Part model, mm, in its own coordinate system. A direction names the side the tool comes from. Give positions to 0.01 mm unless a question says otherwise; leave off trailing zeros. Order: outer loops, then holes, each group sorted by start corner. A loop starts at its lowest first (then second) coordinate and runs counter-clockwise, first axis right, second up. Notation, with made-up numbers: (-27, 73.5) - (15, 73.5) arc R7 ccw to (15, 85.5) - close; hole circle Ø10 at (63, 19.25). An arc over 180 degrees is marked (long way). One line per item, written item: value.
Autodesk Inventor part; units mm, degrees
ref_plane "YZ Plane" through (0, 0, 0) normal (1, 0, 0) x (0, 1, 0)
ref_plane "XZ Plane" through (0, 0, 0) normal (0, 1, 0) x (-1, 0, 0)
ref_plane "XY Plane" through (0, 0, 0) normal (0, 0, 1) x (1, 0, 0)
sketch "Sketch1" plane through (0, 0, 0) normal (0, 1, 0) x (-1, 0, 0)
  circle A0 centre (0, 0) radius 16
  circle A1 centre (0, 0) radius 2.5
  dimension "d0" = 32
  dimension "d1" = 5
extrude "Extrusion1" add sketch "Sketch1" along normal blind 2
sketch "Sketch2" plane through (0, 2, 0) normal (0, 1, 0) x (1, 0, 0)
  circle A0 centre (0, 0) radius 2.5
  circle A1 centre (0, 0) radius 12.5
  dimension "d4" = 25
extrude "Extrusion2" add sketch "Sketch2" along normal blind 3
sketch "Sketch3" plane through (0, 5, 0) normal (0, 1, 0) x (1, 0, 0)
  circle A0 centre (0, 0) radius 16
  circle A1 centre (0, 0) radius 2.5
  dimension "d7" = 32
  dimension "d8" = 5
extrude "Extrusion3" add sketch "Sketch3" along normal blind 2
fillet "Fillet1" radius 0.2 1 edges at (-16, 7, 0)
properties part number "Piston" material "Aluminum 6061"
1) Drop flat-ended pins along their axis: P1, Ø4, axis at x = 9, y = 5.5, coming from the -Z side; P2, Ø4, axis at x = -11, y = 1, coming from the +Z side. Give the stop position or say it passes through.
Answer:
P1: stops at z = -14.39
P2: stops at z = 13.23
2) Two-plate mould, pull along Y, no slides. Class faces 1 (the face through (0, 0, -3)), 2 (the face through (-10, 5, 8)), 3 (the face through (3.47, 0.99, 15.62)): pulls with the +Y half, pulls with the -Y half, needs draft (parallel to the pull), parting line crosses it, or undercut.
Answer:
face 1: pulls with the -Y half
face 2: undercut
face 3: needs draft
3) Which spindle directions (+Z, -Z, +X, -X, +Y, -Y) get a long thin tool onto all of the face, cutting with end or side? Do faces 4 (the face through (0, 7, 3)), 5 (the face through (10, 2, -8)). Say none if no direction does.
Answer:
face 4: +Z, -Z, +X, -X, +Y
face 5: none
4) Slice it at A-A on y = 6. Write the cut outline in (x, z).
Answer:
outline: circle Ø32 at (0, 0); hole circle Ø5 at (0, 0)
5) Wall check: line 1 along X through (y, z) = (3.3, 0); line 2 along X through (y, z) = (6.45, 0). Give the ranges that are in metal, low to high. Write a range as [from, to].
Answer:
line 1: x = [-12.5, -2.5], [2.5, 12.5]
line 2: x = [-16, -2.5], [2.5, 16]
